Model file for the job. Use its own axes, mm. Coordinates: 2 decimals unless noted, no trailing zeros. Order: outer loops, then holes, each group sorted by start corner. A loop starts at its lowest first (then second) coordinate and runs counter-clockwise, first axis right, second up.
from build123d import *

# Parameters (mm, degrees)
F0_W      = 12.7
F0_H      = 12.7
F1_DEPTH  = 88.9
F15_DEPTH = 25.4
F16_DEPTH = 25.4
F17_DEPTH = 25.4
F18_DEPTH = 25.4


with BuildPart() as f1:
    # F0 (on Top) → F1 (new body)
    with BuildSketch(Plane.XY):
        Rectangle(F0_W, F0_H)
    extrude(amount=-F1_DEPTH)

    # F11 (on 3pt) → F15 (cut)
    with BuildSketch(Plane(origin=(-29.3548700028, 29.3548700028, -23.5027056937), x_dir=(-0.7882634225, -0.4803480231, 0.3845862106), z_dir=(-0.615337937, 0.615337937, -0.4926646391))):
        Polygon((-29.1842413909, -69.3975402572), (-29.1842413909, -59.2375402572), (-37.2399240707, -65.4287902572), align=None)
    extrude(amount=F15_DEPTH, mode=Mode.SUBTRACT)

    # F12 (on 3pt) → F16 (cut)
    with BuildSketch(Plane(origin=(-29.3548700028, -29.3548700028, -23.5027056937), x_dir=(0.7882634225, -0.4803480231, -0.3845862106), z_dir=(-0.615337937, -0.615337937, -0.4926646391))):
        Polygon((37.2399240707, -65.4287902572), (29.1842413909, -59.2375402572), (29.1842413909, -69.3975402572), align=None)
    extrude(amount=F16_DEPTH, mode=Mode.SUBTRACT)

    # F13 (on 3pt) → F17 (cut)
    with BuildSketch(Plane(origin=(29.3548700028, -29.3548700028, -23.5027056937), x_dir=(-0.7882634225, -0.4803480231, -0.3845862106), z_dir=(-0.615337937, 0.615337937, 0.4926646391))):
        Polygon((29.1842413909, -59.2375402572), (29.1842413909, -69.3975402572), (37.2399240707, -65.4287902572), align=None)
    extrude(amount=-F17_DEPTH, mode=Mode.SUBTRACT)

    # F14 (on 3pt) → F18 (cut)
    with BuildSketch(Plane(origin=(29.3548700028, 29.3548700028, -23.5027056937), x_dir=(0.7882634225, -0.4803480231, 0.3845862106), z_dir=(-0.615337937, -0.615337937, 0.4926646391))):
        Polygon((-29.1842413909, -69.3975402572), (-29.1842413909, -59.2375402572), (-37.2399240707, -65.4287902572), align=None)
    extrude(amount=-F18_DEPTH, mode=Mode.SUBTRACT)


solid = f1.part
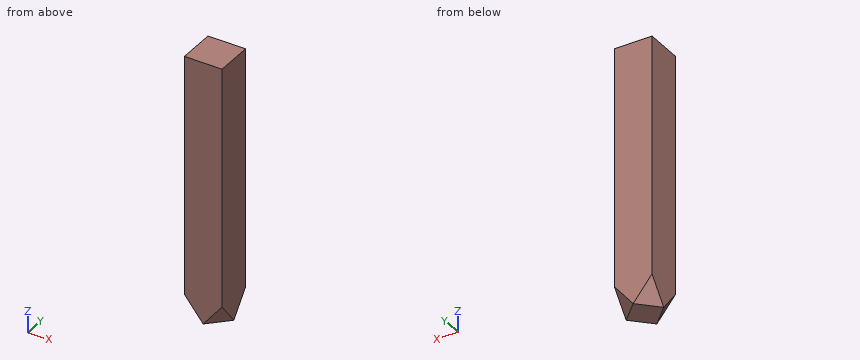
Q1. Probe line 1 (Z direction, x = -2.25, y = -5.25); line 2 (Z direction, x = -3.5, y = 5.75); line 3 (Y direction, x = 3.5, z = -85). List the from-to ranges inside material, lowest first.
Established:
line 1: z = -87.46 to 0
line 2: z = -85.28 to 0
line 3: y = -5.97 to 5.97
Q2. Cut at A-A, the plane y = -5. List the corners of the cut face in (x, z) (3 decimals).
Established:
outline: (-6.35, -82.655) - (-1.35, -88.9) - (1.35, -88.9) - (6.35, -82.655) - (6.35, 0) - (-6.35, 0) - close
Q3. Cut at B-B, the plane y = 4.75. List the corners of the cut face in (x, z), plus the area to 3 significant figures.
Established:
outline: (-6.35, -82.97) - (-1.6, -88.9) - (1.6, -88.9) - (6.35, -82.97) - (6.35, 0) - (-6.35, 0) - close
area: 1,100 mm2
